```python
from build123d import *


with BuildPart() as part:
    # Sweep1: sweep along a path in Sketch2
    with BuildLine(Plane(origin=(0, 0, 0), x_dir=(1, 0, 0), z_dir=(0, 1, 0))) as sweep1_path:
        Line((104.841229183, 1.25), (9.921567416, 1.25))
        ThreePointArc((9.921567416, 1.25), (6.386033511, 1.895856533), (3.307189139, 3.75))
        ThreePointArc((3.307189139, 3.75), (-5, 0), (3.307189139, -3.75))
        ThreePointArc((3.307189139, -3.75), (6.386033511, -1.895856533), (9.921567416, -1.25))
        Line((9.921567416, -1.25), (104.841229183, -1.25))
    # Sketch3 → Sweep1 (sweep)
    with BuildSketch(Plane.ZY.offset(-104.841229183)):
        with BuildLine():
            Line((1.25, 2.291287847), (1.25, -2.291287847))
            ThreePointArc((1.25, -2.291287847), (4.75, 0), (1.25, 2.291287847))
        make_face()
    sweep(path=sweep1_path.line)


solid = part.part
```
Here's how the part is built. I have some questions about the finished solid (model axes, mm). A direction names the side the tool comes from. Coordinates: 2 decimals unless noted, no trailing zeros. Order: outer loops, then holes, each group sorted by start corner. A loop starts at its lowest first (then second) coordinate and runs counter-clockwise, first axis right, second up.
1) Imagine slicing it at C-C on z = 0. List the corners of the cut face in (x, y) for me, and give its area (3 significant figures).
2) Imagine slicing it at A-A on x = 82. List the corners of the cut face in (y, z) for me.
3) I need wall thicknesses on line 1 (Y direction, x = 57.5, z = 2.5); line 2 (Z direction, x = 0, y = -0.75); line 3 (X direction, y = 1.95, z = -2.5). Which ranges of each line are inside material? Lowest first, please.
4) Will these pins go through, and if not, where does the flat tip stop? pin 1 (1.4 mm diameter, centred on x = 51.5, y = -0.5, fed in from -Z); pin 2 (1 mm diameter, centred on y = -1.5, z = -1.5, fed in from -X); pin 3 (2 mm diameter, centred on x = 69.5, y = -0.5, fed in from +Z); pin 4 (9 mm diameter, centred on x = 0, z = 0, fed in from -Y).
5) We'd pull the mould along X, two halves only. Please class faces 1 (the face through (104.841, 0, -3)), 2 (the face through (57, 0, -1.25)), 3 (the face through (-5, 0, 0)), 4 (the face through (6.43, -0.03, -1.88)): +X half, -X half, draft (parallel to the pull), parting line (faces both ways), or undercut.
6) Imagine slicing it at B-B on y = 0. List the corners of the cut face in (x, z) for me (3 decimals).
7) Which directions (+Z, -Z, +X, -X, +Y, -Y) give clear straight access to the entire face, cutting with the end or side of a thin tool? Please do faces 5 (the face through (104.841, 0, 3)), 6 (the face through (6.339, -0.032, 1.914)), 7 (the face through (58.05, 0.07, 4.75)), 8 (the face through (58, 0, 1.25)).
Response values:
1. outline: (-5, -2.29) - (-5, 2.29) arc R2.5 ccw (long way) to start
1. area: 14.7 mm2
2. outline: (-2.29, -1.25) arc R2.5 ccw (long way) to (2.29, -1.25) - close; (-2.29, 1.25) - (2.29, 1.25) arc R2.5 ccw (long way) to start
3. line 1: y = -2.49 to 2.49
3. line 2: z = -8.38 to -5, 5 to 8.38
3. line 3: x = -7.14 to -4.33, 5.08 to 104.84
4. pin 1: stops at z = -4.75
4. pin 2: stops at x = -8.17
4. pin 3: stops at z = 4.75
4. pin 4: passes through
5. face 1: +X half
5. face 2: draft
5. face 3: undercut
5. face 4: undercut
6. outline: (3.307, -3.75) arc R5 cw (long way) to (3.307, 3.75) arc R10 ccw to (9.922, 1.25) - (104.841, 1.25) - (104.841, 4.75) - (9.922, 4.75) arc R6.5 cw to (5.622, 6.375) arc R8.5 ccw (long way) to (5.622, -6.375) arc R6.5 cw to (9.922, -4.75) - (104.841, -4.75) - (104.841, -1.25) - (9.922, -1.25) arc R10 ccw to start
7. face 5: +Z, -Z, +X, +Y, -Y
7. face 6: +Y, -Y
7. face 7: +X
7. face 8: +X, +Y, -Y
